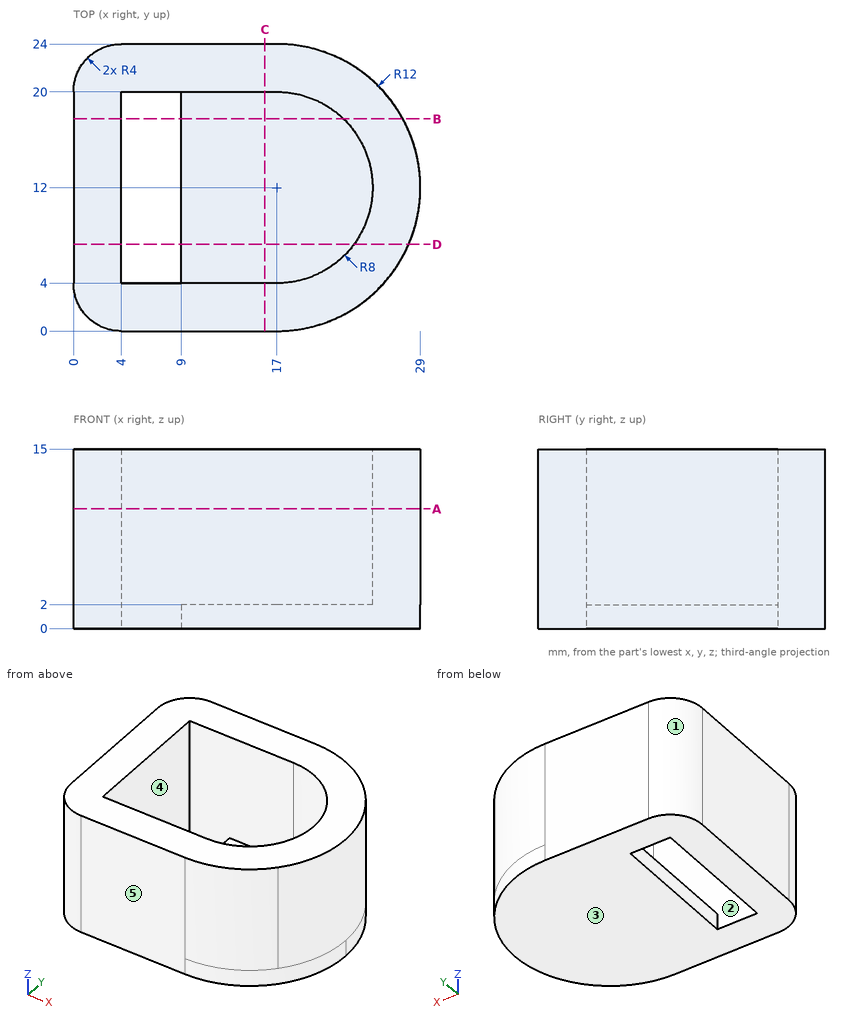
Geometry check sheet. Reference: drawing and pictorial views, mm from the part's lowest x, y, z. A direction names the side the tool comes from. Give positions to 0.01 mm unless a question says otherwise; leave off trailing zeros. Order: outer loops, then holes, each group sorted by start corner. A loop starts at its lowest first (then second) coordinate and runs counter-clockwise, first axis right, second up. Notation, with made-up numbers: (58, -26.75) - (96, -26.75) arc R24 ccw to (96, -7.75) - close; hole circle Ø3 at (83, -14). An arc over 180 degrees is marked (long way). Use one line per item in the form item = value.
1) Sectioned sample at B-B (y = 17.75). Record the boundary of the cut face in (x, z).
Working result:
outline = (0, 0) - (4, 0) - (4, 15) - (0, 15) - close; (9, 0) - (27.53, 0) - (27.53, 15) - (22.56, 15) - (22.56, 2) - (9, 2) - close
2) Material ranges on probe 1 along Y at (x, z) = (5.5, 11); probe 2 along X at (y, z) = (11.75, 1.5); probe 3 along X at (y, z) = (18.5, 3.25), recorded low to high. Write a range as from..to.
Working result:
probe_1 = 0..4, 20..24
probe_2 = 0..4, 9..29
probe_3 = 0..4, 21.66..27.09
3) Sectioned sample at D-D (y = 7.25). Record the boundary of the cut face in (x, z).
Working result:
outline = (0, 0) - (4, 0) - (4, 15) - (0, 15) - close; (9, 0) - (28.02, 0) - (28.02, 15) - (23.44, 15) - (23.44, 2) - (9, 2) - close
4) Depth check by flat-ended pin: pin 1 Ø1.5 at (x, y) = (7.5, 7) entering from -Z; pin 2 Ø5 at (x, z) = (21.5, 4.5) entering from -Y; pin 3 Ø5 at (x, y) = (18, 11) entering from +Z; pin 4 Ø2 at (y, z) = (9.5, 12) entering from +X. Enter the tip coordinate at first touch or a pass-through.
Working result:
pin_1 = through
pin_2 = 0.17
pin_3 = 2
pin_4 = 28.91
5) Sectioned sample at A-A (z = 10). Record the boundary of the cut face in (x, y), and give its area (3 significant figures).
Working result:
outline = (0, 4) arc R4 ccw to (4, 0) - (17, 0) arc R12 ccw to (17, 24) - (4, 24) arc R4 ccw to (0, 20) - close; hole (4, 4) - (17, 4) arc R8 ccw to (17, 20) - (4, 20) - close
area = 319 mm^2
6) Access from +Z, -Z, +X, -X, +Y, -Y to the whole of each face (thin tool, end or side, straight path). Record for the marked faces 1 and 2.
Working result:
face_1 = +Z, -Z, -X, +Y
face_2 = +Z
7) Draft check along Y on the marked faces 3, 4 and 5. Enter one of: released by +Y, released by -Y, zero draft, split by the parting line, or undercut.
Working result:
face_3 = zero draft
face_4 = undercut
face_5 = released by -Y
8) Sectioned sample at C-C (x = 16). Record the boundary of the cut face in (y, z), and give its area (3 significant figures).
Working result:
outline = (0, 0) - (24, 0) - (24, 15) - (20, 15) - (20, 2) - (4, 2) - (4, 15) - (0, 15) - close
area = 152 mm^2
